Autodesk Fusion 360 part; units mm, degrees
sketch "Bracket" plane through (0, 0, 0) normal (1, 0, 0) x (0, 1, 0)
  line L0 (0, 0) -> (2, 0)
  line L1 (2, -2) -> (2, -200)
  line L2 (2, -200) -> (0, -200)
  line L3 (0, -200) -> (0, 0)
  line L4 (0, 0) -> (120, 0)
  line L5 (120, 0) -> (120, -2)
  line L6 (120, -2) -> (2, -2)
  line L7 (0, -2) -> (0, 0)
  dimension "d1" = 2
  dimension "d2" = 200
  dimension "d3" = 120
  dimension "d4" = 2
extrude "Extrude1" add sketch "Bracket" along normal blind 18
fillet "Fillet1" radius 3 1 edges at (9, 2, -2)
fillet "Fillet2" radius 4 1 edges at (9, 0, 0)
sketch "Front Holes" plane through (0, 0, 0) normal (0, -1, 0) x (1, 0, 0)
  line L0 (18, -4) -> (0, -4)
  line L1 (0, -4) -> (0, -200)
  line L2 (0, -200) -> (18, -200)
  line L3 (18, -200) -> (18, -4)
  line L4 (9, -200) -> (9, -113.9355) construction
  circle A0 centre (9, -187) radius 2.25
  circle A1 centre (9, -155) radius 2.25
  circle A2 centre (9, -127) radius 2.25
  dimension "d9" = 4.5
  dimension "d10" = 4.5
  dimension "d11" = 4.5
  dimension "d12" = 13
  dimension "d13" = 32
  dimension "d14" = 28
sketch "Top Holes" plane through (0, 0, 0) normal (0, 0, 1) x (-1, 0, 0)
  line L0 (0, -4) -> (-18, -4)
  line L1 (-18, -4) -> (-18, -120)
  line L2 (-18, -120) -> (0, -120)
  line L3 (0, -120) -> (0, -4)
  line L4 (-9, -120) -> (-9, -16.6564) construction
  circle A0 centre (-9, -102) radius 1.75
  circle A1 centre (-9, -79) radius 1.75
  dimension "d15" = 3.5
  dimension "d16" = 3.5
  dimension "d17" = 18
  dimension "d18" = 23
extrude "Extrude2" cut sketch "Front Holes" against normal blind 5 contours A0 | A1 | A2
extrude "Extrude3" cut sketch "Top Holes" against normal blind 5 contours A0 | A1
equation "d10 = d9"
equation "d11 = d9"
equation "d16 = d15"
Check sheet for the modelled part. Datum: model origin and axes. Units: mm. A direction names the side the tool comes from. Give positions to 0.01 mm unless a question says otherwise; leave off trailing zeros. Write each loop counter-clockwise with the first axis right and the second up, starting at its lowest first coordinate (ties: lowest second). Pieces come first, ordered by that corner, then holes. Notation, with made-up numbers: (26.5, -2) -> (67.5, -2) arc R22 cw to (67.5, 24) -> close; hole circle Ø11 at (71, 57.25). An arc over 180 degrees is marked (long way). Use CSV: the item, a comma, the result in double quotes. Start each with the question number.
Q1. Cross-section at C-C on y = 32. Enter the section's corners in (x, z).
Q2. Scan lines: line 1 along X through (y, z) = (0.6, -187); line 2 along X through (y, z) = (79, -0.9); line 3 along Z through (x, y) = (9, 1.1) (3 decimals). Record each from-to range of solid material in increasing order.
Q3. Depth check by flat-ended pin: P1, Ø6, axis at x = 9, z = -127, coming from the +Y side; P2, Ø9, axis at x = 8, y = 81.5, coming from the -Z side. Enter the tip coordinate at first touch or a pass-through.
Q4. Cross-section at A-A on z = -187. Enter the section's corners in (x, y).
Q5. Cross-section at B-B on x = 2.25. Enter the section's corners in (y, z), and give its area (3 significant figures).
Q6. Release check for a two-part mould opening along X. For faces 1 (the cylindrical face through (8.512, 0.986, -157.196)), 2 (the cylindrical face through (9.126, 1.203, -1.141)) record: +X half, -X half, draft (parallel to the pull), parting line (faces both ways), or undercut.
Q7. Tool access check on faces 3 (the cylindrical face through (8.512, 0.986, -189.196)), 4 (the flat face through (9, 2, -101)). Record the directions out of +Z, -Z, +X, -X, +Y, -Y that give a thin tool (end or side, any length) a straight path to the whole face; none if there is none.
Working result:
1,outline,"(0, -2) -> (18, -2) -> (18, 0) -> (0, 0) -> close"
2,line 1,"x = 0 to 6.75, 11.25 to 18"
2,line 2,"x = 0 to 7.25, 10.75 to 18"
2,line 3,"z = -200 to -189.25, -184.75 to -157.25, -152.75 to -129.25, -124.75 to -1.245"
3,P1,"stops at y = 2"
3,P2,"stops at z = -2"
4,outline,"(0, 0) -> (6.75, 0) -> (6.75, 2) -> (0, 2) -> close; (11.25, 0) -> (18, 0) -> (18, 2) -> (11.25, 2) -> close"
5,outline,"(0, -200) -> (2, -200) -> (2, -5) arc R3 cw to (5, -2) -> (120, -2) -> (120, 0) -> (4, 0) arc R4 ccw to (0, -4) -> close"
5,area,"634 mm^2"
6,face 1,"undercut"
6,face 2,"draft"
7,face 3,"+Y, -Y"
7,face 4,"-Z, +X, -X, +Y"
